Source: CAD feature listing. Evaluate the final solid. Frame: model axes, mm. A direction names the side the tool comes from. Give positions to 0.01 mm unless a question says otherwise; leave off trailing zeros. Write each loop counter-clockwise with the first axis right and the second up, starting at its lowest first coordinate (ties: lowest second). Pieces come first, ordered by that corner, then holes. Notation, with made-up numbers: (-14.5, -13.75) -> (40.5, -13.75) arc R10 cw to (40.5, -0.75) -> close; hole circle Ø7 at (-36.5, -31.5). An arc over 180 degrees is marked (long way). Answer as a JSON object with one key per item and string values. Group by question number.
Item 1: Access query for faces 4 (the face through (1.325, -1.493, -1.277)), 5 (the face through (1, 2.2, 1)), 6 (the face through (0.91, -0.49, -0.06)), 7 (the face through (1.002, 1.461, 0.121)). Directions: +Z, -Z, +X, -X, +Y, -Y. A direction counts if a zero-diameter tool reaches every point of the face in a straight line with its end or side. Return the directions, or none.
Item 2: Pull-direction query (Y, two-part tool) for faces 1 (the face through (-1, 0.7, -1)), 2 (the face through (-1.17, 1.08, 2.42)), 3 (the face through (1, 0, 1)); classes: pulls with the +Y half, pulls with the -Y half, needs draft (parallel to the pull), parting line crosses it, or undercut.
Item 3: Section query A-A on x = 0.2. Return the cut outline in (y, z).
Item 4: Section query B-B on z = -0.65. Return the cut outline in (x, y).
Item 5: Section query D-D on y = 1.5. Return the cut outline in (x, z), plus the area to 3 significant figures.
Item 6: Section query C-C on y = -1.5. Return the cut outline in (x, z), plus the area to 3 significant figures.
Item 7: First-contact query: pin 1 Ø2 at (x, y) = (1, -3.5) entering from +Z. Flat tip, straight axial feed; report the tip coordinate or a pass-through.
Item 8: Ray query, probe 1 along Y at (x, z) = (1.4, -0.45); probe 2 along Y at (x, z) = (0.7, 1.65); probe 3 along Y at (x, z) = (-1.95, -0.55). Return the intervals inside material, ascending. Write a range as from..to.
from build123d import *

# Parameters (mm, degrees)
SKETCH1_R           = 3
BOSS_EXTRUDE1_DEPTH = 2.2
SKETCH1_3_R         = 1.6
BOSS_EXTRUDE2_DEPTH = 1
SKETCH5_R           = 1.5
BOSS_EXTRUDE3_DEPTH = 1
SKETCH6_R           = 2
BOSS_EXTRUDE4_DEPTH = 1
SKETCH8_R           = 1.5
BOSS_EXTRUDE5_DEPTH = 3.5
SKETCH10_R          = 1.8
BOSS_EXTRUDE6_DEPTH = 1
SKETCH12_R          = 1.65
CUT_EXTRUDE1_DEPTH  = 1.5


with BuildPart() as part:
    # Sketch1 → Boss-Extrude1 (new body)
    with BuildSketch(Plane(origin=(0, 0, 0), x_dir=(1, 0, 0), z_dir=(0, 1, 0))):
        with Locations((-0.522013312, 0.511138034)):
            Circle(SKETCH1_R)
    extrude(amount=BOSS_EXTRUDE1_DEPTH)

    # Sketch1<3> → Boss-Extrude2 (add)
    with BuildSketch(Plane(origin=(0, 0, 0), x_dir=(1, 0, 0), z_dir=(0, 1, 0))):
        with Locations((-0.522013312, 0.511138034)):
            Circle(SKETCH1_3_R)
    extrude(amount=BOSS_EXTRUDE2_DEPTH)

    # Sketch5 → Boss-Extrude3 (add)
    with BuildSketch(Plane.XZ):
        with Locations((-0.522013312, -0.511138034)):
            Circle(SKETCH5_R)
    extrude(amount=BOSS_EXTRUDE3_DEPTH)

    # Sketch6 → Boss-Extrude4 (add)
    with BuildSketch(Plane.XZ.offset(1)):
        with Locations((-0.522013312, -0.511138034)):
            Circle(SKETCH6_R)
    extrude(amount=BOSS_EXTRUDE4_DEPTH)

    # Sketch8 → Boss-Extrude5 (add)
    with BuildSketch(Plane(origin=(0, -2, 0), x_dir=(-1, 0, 0), z_dir=(0, -1, 0))):
        with Locations((0.522013312, 0.511138034)):
            Circle(SKETCH8_R)
    extrude(amount=BOSS_EXTRUDE5_DEPTH)

    # Sketch10 → Boss-Extrude6 (add)
    with BuildSketch(Plane.XZ.offset(5.5)):
        with Locations((-0.522013312, -0.511138034)):
            Circle(SKETCH10_R)
    extrude(amount=-BOSS_EXTRUDE6_DEPTH)

    # Sketch12 → Cut-Extrude1 (cut)
    with BuildSketch(Plane(origin=(0, 2.2, 0), x_dir=(1, 0, 0), z_dir=(0, 1, 0))):
        with Locations((-0.522013312, 0.511138034)):
            Circle(SKETCH12_R)
    extrude(amount=-CUT_EXTRUDE1_DEPTH, mode=Mode.SUBTRACT)


solid = part.part
Worked answers:
{
 "1": {"face 4": "-Y", "face 5": "+Z, -Z, +X, -X, +Y", "face 6": "none", "face 7": "+Y"},
 "2": {"face 1": "pulls with the +Y half", "face 2": "needs draft", "face 3": "undercut"},
 "3": {"outline": "(-5.5, -2.16) -> (-4.5, -2.16) -> (-4.5, -1.83) -> (-2, -1.83) -> (-2, -2.38) -> (-1, -2.38) -> (-1, -1.83) -> (0, -1.83) -> (0, -3.42) -> (2.2, -3.42) -> (2.2, -1.99) -> (0.7, -1.99) -> (0.7, 0.97) -> (2.2, 0.97) -> (2.2, 2.4) -> (0, 2.4) -> (0, 0.8) -> (-1, 0.8) -> (-1, 1.35) -> (-2, 1.35) -> (-2, 0.8) -> (-4.5, 0.8) -> (-4.5, 1.14) -> (-5.5, 1.14) -> close"},
 "4": {"outline": "(-3.52, 0) -> (-2.02, 0) -> (-2.02, -1) -> (-2.52, -1) -> (-2.52, -2) -> (-2.02, -2) -> (-2.02, -4.5) -> (-2.32, -4.5) -> (-2.32, -5.5) -> (1.27, -5.5) -> (1.27, -4.5) -> (0.97, -4.5) -> (0.97, -2) -> (1.47, -2) -> (1.47, -1) -> (0.97, -1) -> (0.97, 0) -> (2.47, 0) -> (2.47, 2.2) -> (1.12, 2.2) -> (1.12, 0.7) -> (-2.17, 0.7) -> (-2.17, 2.2) -> (-3.52, 2.2) -> close"},
 "5": {"outline": "circle Ø6 at (-0.52, -0.51); hole circle Ø3.3 at (-0.52, -0.51)", "area": "19.7 mm^2"},
 "6": {"outline": "circle Ø4 at (-0.52, -0.51)", "area": "12.6 mm^2"},
 "7": {"pin 1": "z = 0.9"},
 "8": {"probe 1": "-2..-1, 0..2.2", "probe 2": "0..2.2", "probe 3": "-5.5..0.7"}
}
